For this review, take the finished solid that the model builds, in its own axes (mm). A direction names the side the tool comes from. Coordinates: 2 decimals unless noted, no trailing zeros. Write each loop counter-clockwise with the first axis right and the second up, starting at its lowest first coordinate (ties: lowest second). Pieces come first, ordered by that corner, then holes. Notation, with made-up numbers: (5.5, -28.75) - (40.5, -28.75) arc R23 ccw to (40.5, 10.25) - close; hole circle Ø6 at (-15, 16.25). An arc over 180 degrees is marked (long way). Write each question's results on one line, items separated by ' | '.
from build123d import *

# Parameters (mm, degrees)
BOSS_EXTRUDE1_START = 19
SKETCH2_R           = 4.5
SKETCH2_R_2         = 4
BOSS_EXTRUDE1_DEPTH = 1


with BuildPart() as part:
    # Sketch2 → Boss-Extrude1 (new body)
    with BuildSketch(Plane.XY.offset(BOSS_EXTRUDE1_START)):
        with BuildLine():
            Line((55, 0), (45.421564163, -1.006734174))
            ThreePointArc((45.421564163, -1.006734174), (39, -6.5), (32.578435837, -1.006734174))
            Line((32.578435837, -1.006734174), (7.101007974, -3.684519746))
            ThreePointArc((7.101007974, -3.684519746), (-8, 0), (7.101007974, 3.684519746))
            Line((7.101007974, 3.684519746), (32.578435837, 1.006734174))
            ThreePointArc((32.578435837, 1.006734174), (39, 6.5), (45.421564163, 1.006734174))
            Line((45.421564163, 1.006734174), (55, 0))
        make_face()
        Circle(SKETCH2_R, mode=Mode.SUBTRACT)
        with Locations((40, 0)):
            Circle(SKETCH2_R_2, mode=Mode.SUBTRACT)
    extrude(amount=BOSS_EXTRUDE1_DEPTH)


solid = part.part
Q1. Take a section at C-C on x = 12.5. State the section outline as (y, z) points.
Results found:
outline: (-3.12, 19) - (3.12, 19) - (3.12, 20) - (-3.12, 20) - close
Q2. Take a section at A-A on z = 19.8. State the section outline as (x, y) points.
Results found:
outline: (7.1, -3.68) - (32.58, -1.01) arc R6.5 ccw to (45.42, -1.01) - (55, 0) - (45.42, 1.01) arc R6.5 ccw to (32.58, 1.01) - (7.1, 3.68) arc R8 ccw (long way) to start; hole circle Ø9 at (0, 0); hole circle Ø8 at (40, 0)
Q3. Mouldability with a two-part tool opening along Y and no side actions: class faces 1 (the face through (50.278, -0.496, 19.493)), 2 (the face through (17, -1, 19)), 3 (the face through (36.8, -2.4, 19.5)) as pulls with the +Y half, pulls with the -Y half, needs draft (parallel to the pull), parting line crosses it, or undercut.
Results found:
face 1: pulls with the -Y half | face 2: needs draft | face 3: undercut
Q4. For faces 4 (the face through (19.661, 2.364, 19.493)), 5 (the face through (-0.59, 4.46, 19.49)), 6 (the face through (20.018, -2.327, 19.493)), list the 3-axis set-ups (+Z, -Z, +X, -X, +Y, -Y) from which the entire face can be reached by the end or side of a thin tool; tool diameter is ignored.
Results found:
face 4: +Z, -Z, +Y | face 5: +Z, -Z | face 6: +Z, -Z, -Y
Q5. Take a section at B-B on x = 0. State the section outline as (y, z) points, plus the area to 3 significant figures.
Results found:
outline: (-8, 19) - (-4.5, 19) - (-4.5, 20) - (-8, 20) - close; (4.5, 19) - (8, 19) - (8, 20) - (4.5, 20) - close | area: 7.00 mm2
Q6. Wall thickness on line 1 along Y through (x, z) = (0, 19.45); line 2 along X through (y, z) = (5, 19.1) (3 decimals); line 3 along Y through (x, z) = (40, 19.6): over which ranges is each line inside the solid? List them lowest first. Write a range as from..to.
Results found:
line 1: -8..-4.5, 4.5..8 | line 2: -6.245..6.245, 34.847..43.153 | line 3: -6.42..-4, 4..6.42
